```python
from build123d import *

# Parameters (mm, degrees)
EXTRUDE_1_DEPTH          = 5.5
SKETCH_5_R               = 7
CUT_EXTRUDE_1_DEPTH      = 316.527538037
SKETCH_6_R               = 1.55
CUT_EXTRUDE_2_DEPTH      = 316.527538037
PATTERN_CIRCULAR_1_COUNT = 3
SKETCH_7_W               = 7.5
SKETCH_7_H               = 20
CUT_EXTRUDE_3_DEPTH      = 316.527538037
SKETCH_8_W               = 7.5
SKETCH_8_H               = 20
CUT_EXTRUDE_4_DEPTH      = 316.6542844
CUT_EXTRUDE_5_DEPTH      = 316.6542844
CUT_EXTRUDE_6_DEPTH      = 316.6542844


with BuildPart() as part:
    # ｽｹｯﾁ1 → ﾎﾞｽ - 押し出し1 (new body)
    with BuildSketch(Plane.XY):
        with BuildLine():
            Line((0, 0), (0, 300))
            Line((0, 300), (50, 270))
            Line((50, 270), (97.608284791, 0))
            ThreePointArc((97.608284791, 0), (48.804142396, -48.804142396), (0, 0))
        make_face()
    extrude(amount=EXTRUDE_1_DEPTH)

    # ｽｹｯﾁ5 → ｶｯﾄ - 押し出し1 (cut, through all)
    with BuildSketch(Plane(origin=(0, 0, 0), x_dir=(-1, 0, 0), z_dir=(0, 0, -1))):
        with Locations((-25, 261.643590902)):
            Circle(SKETCH_5_R)
    extrude(amount=-CUT_EXTRUDE_1_DEPTH, mode=Mode.SUBTRACT)

    # ｽｹｯﾁ6 → ｶｯﾄ - 押し出し2 (cut, through all)
    with BuildSketch(Plane(origin=(0, 0, 0), x_dir=(-1, 0, 0), z_dir=(0, 0, -1))):
        with Locations((-15.5, 261.643590902)):
            Circle(SKETCH_6_R)
    cut_extrude_2 = extrude(amount=-CUT_EXTRUDE_2_DEPTH, mode=Mode.SUBTRACT)

    # 円形ﾊﾟﾀｰﾝ1: ｶｯﾄ - 押し出し2 ×3 about axis
    pattern_circular_1_axis = Axis((25, 261.643590902, 0), (0, 0, 1))
    for i in range(1, PATTERN_CIRCULAR_1_COUNT):
        add(cut_extrude_2.rotate(pattern_circular_1_axis, i * 360 / PATTERN_CIRCULAR_1_COUNT), mode=Mode.SUBTRACT)

    # ｽｹｯﾁ7 → ｶｯﾄ - 押し出し3 (cut, through all)
    with BuildSketch(Plane(origin=(0, 0, 0), x_dir=(-1, 0, 0), z_dir=(0, 0, -1))):
        with Locations((-3.75, 14.792318117)):
            Rectangle(SKETCH_7_W, SKETCH_7_H)
    extrude(amount=-CUT_EXTRUDE_3_DEPTH, mode=Mode.SUBTRACT)

    # ｽｹｯﾁ8 → ｶｯﾄ - 押し出し4 (cut, through all)
    with BuildSketch(Plane(origin=(0, 0, -5), x_dir=(-1, 0, 0), z_dir=(0, 0, -1))):
        with Locations((-3.75, 241.643590902)):
            Rectangle(SKETCH_8_W, SKETCH_8_H)
    extrude(amount=-CUT_EXTRUDE_4_DEPTH, mode=Mode.SUBTRACT)

    # ｽｹｯﾁ9 → ｶｯﾄ - 押し出し5 (cut, through all)
    with BuildSketch(Plane(origin=(0, 0, -5), x_dir=(-1, 0, 0), z_dir=(0, 0, -1))):
        Polygon((-96.736481777, 4.944240587), (-93.263518223, 24.640395647), (-87.5, 23.624131881), (-87.5, 3.315599643), align=None)
    extrude(amount=-CUT_EXTRUDE_5_DEPTH, mode=Mode.SUBTRACT)

    # ｽｹｯﾁ10 → ｶｯﾄ - 押し出し6 (cut, through all)
    with BuildSketch(Plane(origin=(0, 0, -5), x_dir=(-1, 0, 0), z_dir=(0, 0, -1))):
        Polygon((-53.263518223, 251.491668432), (-56.736481777, 231.795513372), (-47.5, 230.166872428), (-47.5, 250.475404665), align=None)
    extrude(amount=-CUT_EXTRUDE_6_DEPTH, mode=Mode.SUBTRACT)


solid = part.part
```
For this review, take the finished solid that the model builds, in its own axes (mm). A direction names the side the tool comes from. Round coordinates to 2 decimals unless told otherwise and drop trailing zeros. Write each loop counter-clockwise with the first axis right and the second up, starting at its lowest first coordinate (ties: lowest second). Pieces come first, ordered by that corner, then holes. Notation, with made-up numbers: M 81,40.5 L 115,40.5 A23 ccw 115,59.5 Z; hole C -16,-26 d4. An arc over 180 degrees is marked long. One line per item, written item: value. Start each with the question number.
(1) Insertion check: pin 1 (4 mm diameter, centred on x = 29.75, y = 253.42, fed in from +Z); pin 2 (3 mm diameter, centred on x = 3.5, z = 3.5, fed in from +Y); pin 3 (1.6 mm diameter, centred on y = 238.5, z = 4, fed in from +X); pin 4 (3 mm diameter, centred on x = 2, z = 4, fed in from -Y). Each pin has a flat end and moves straight along its axis. Give the tip position at first contact, or say it passes through.
(2) We need section C-C (x = 10.5). Give the boundary of the cut face in (y, z).
(3) We need section D-D (y = 151). Give the boundary of the cut face in (x, z), and give its area (3 significant figures).
(4) We need section B-B (x = 25). Give the boundary of the cut face in (y, z), and give its area (3 significant figures).
(5) We need section A-A (z = 2.45). Give the boundary of the cut face in (x, y) (3 decimals), and give its area (3 significant figures).
(6) Machinability: for faces 1 (the flat face through (92.054, 4.119, 2.712)), 2 (the flat face through (50.341, 250.976, 2.712)), 3 (the flat face through (7.5, 15, 3)), which of the approach directions +Z, -Z, +X, -X, +Y, -Y give a long, thin tool a straight path to every point of the face, cutting with its end or side? Answer none if there is none.
(7) The part is to be moulded in two halves that separate along Y. For faces 4 (the flat face through (0, 127, 3)), 5 (the flat face through (4, 231.644, 3)), 6 (the flat face through (51.61, 260.88, 2.71)), say which applies: released by +Y, released by -Y, zero draft, split by the parting line, or undercut.
(8) Wall thickness on line 1 (Y direction, x = 29.75, z = 3.3); line 2 (Y direction, x = 15.5, z = 3.85); line 3 (X direction, y = 13.5, z = 0.7): over which ranges is each line inside the solid? List them lowest first.
Result:
1. pin 1: z = 5.5
1. pin 2: y = 298.8
1. pin 3: x = 47.5
1. pin 4: y = -18.15
2. outline: M -30.24,0 L 293.7,0 L 293.7,5.5 L -30.24,5.5 Z
3. outline: M 0,0 L 70.98,0 L 70.98,5.5 L 0,5.5 Z
3. area: 390 mm²
4. outline: M -42.61,0 L 254.64,0 L 254.64,5.5 L -42.61,5.5 Z; M 268.64,0 L 285,0 L 285,5.5 L 268.64,5.5 Z
4. area: 1,720 mm²
5. outline: M 0,0 A48.804 ccw 97.608,0 L 96.736,4.944 L 87.5,3.316 L 87.5,23.624 L 93.264,24.64 L 56.736,231.796 L 47.5,230.167 L 47.5,250.475 L 53.264,251.492 L 50,270 L 0,300 L 0,251.644 L 7.5,251.644 L 7.5,231.644 L 0,231.644 L 0,24.792 L 7.5,24.792 L 7.5,4.792 L 0,4.792 Z; hole C 15.5,261.644 d3.1; hole C 25,261.644 d14; hole C 29.75,253.416 d3.1; hole C 29.75,269.871 d3.1
5. area: 23,600 mm²
6. face 1: +Z, -Z
6. face 2: +Z, -Z, +X
6. face 3: +Z, -Z, -X
7. face 4: zero draft
7. face 5: undercut
7. face 6: released by +Y
8. line 1: -44.93 to 251.87, 254.97 to 256.5, 266.79 to 268.32, 271.42 to 282.15
8. line 2: -35.67 to 260.09, 263.19 to 290.7
8. line 3: 7.5 to 87.5
